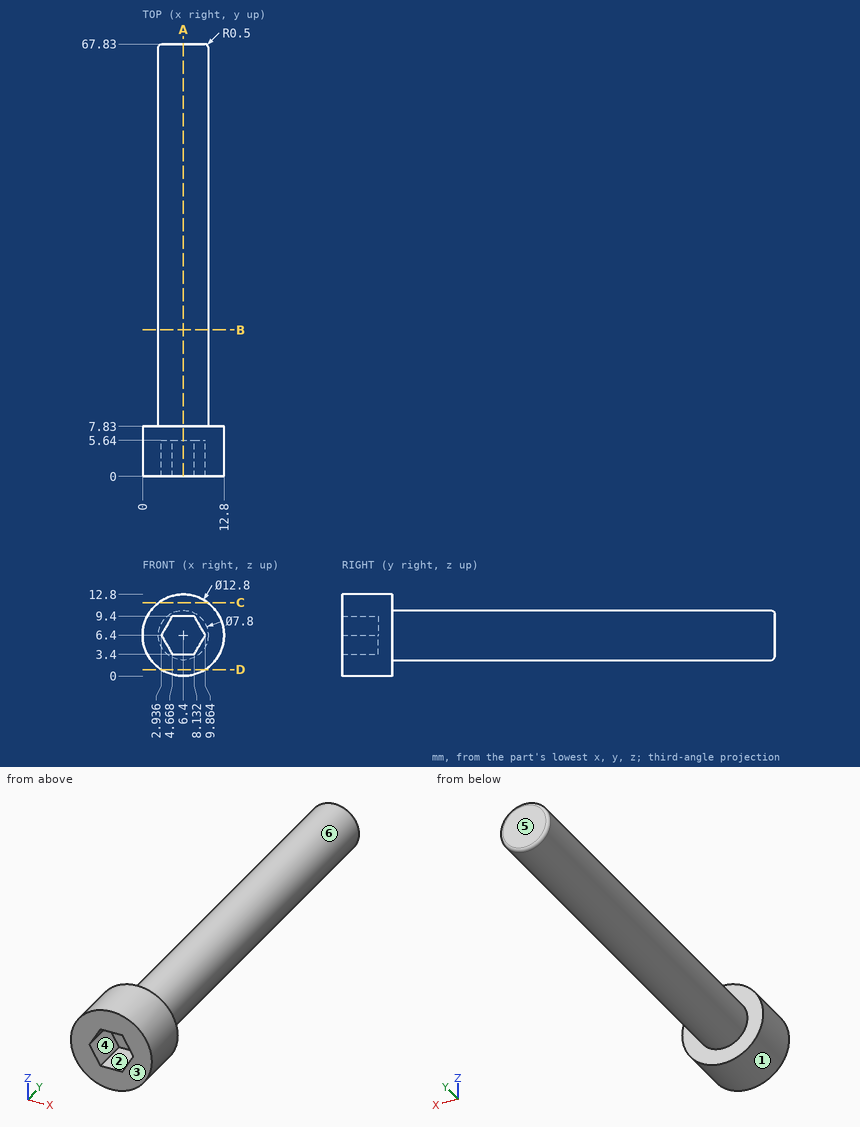
Answer from the drawing. Dimensions are ordinates in mm from the lowest x, y and z of the part. A direction names the side the tool comes from. Round coordinates to 2 decimals unless told otherwise and drop trailing zeros. Loops run counter-clockwise (first coordinate to the right, second up) from the corner with the lowest first, then second, coordinate; pieces in that order, holes last.
1) Consider line 1 (Y direction, x = 11.25, z = 6.5); line 2 (Z direction, x = 9.75, y = 5); line 3 (Y direction, x = 4.75, z = 6.5). Determine where each line is inside the solid, lowest interval first.
Outcome:
line 1: y = 0 to 7.83
line 2: z = 0.95 to 6.2, 6.6 to 11.85
line 3: y = 5.64 to 67.83
2) A cutting plane is placed at B-B on y = 23. Determine the outline of the cut face in (x, z).
Outcome:
outline: circle Ø7.8 at (6.4, 6.4)
3) A cutting plane is placed at D-D on z = 1. Determine the outline of the cut face in (x, y) (3 decimals), plus the area to 3 significant figures.
Outcome:
outline: (2.965, 0) - (9.835, 0) - (9.835, 7.83) - (2.965, 7.83) - close
area: 53.8 mm2
4) A cutting plane is placed at A-A on x = 6.4. Determine the outline of the cut face in (y, z).
Outcome:
outline: (0, 0) - (7.83, 0) - (7.83, 2.5) - (67.33, 2.5) arc R0.5 ccw to (67.83, 3) - (67.83, 9.8) arc R0.5 ccw to (67.33, 10.3) - (7.83, 10.3) - (7.83, 12.8) - (0, 12.8) - (0, 9.4) - (5.64, 9.4) - (5.64, 3.4) - (0, 3.4) - close
5) For the marked faces 5 and 6, determine the directions among +Z, -Z, +X, -X, +Y, -Y from which every point of the face is accessible in a straight line to the end or side of a thin tool.
Outcome:
face 5: +Z, -Z, +X, -X, +Y
face 6: +Y
6) Given P1, Ø2, axis at y = 56.5, z = 5, coming from the -X side, flat-ended and moving along its own axis, determine where the tip first touches the part or whether it passes through.
Outcome:
P1: stops at x = 2.52
7) A cutting plane is placed at C-C on z = 11.5. Determine the outline of the cut face in (x, y).
Outcome:
outline: (2.53, 0) - (10.27, 0) - (10.27, 7.83) - (2.53, 7.83) - close
8) For a pull along X with two mould halves and no side action, classify the marked faces 1, 2, 3 and 4 as released by +X, released by -X, zero draft, split by the parting line, or undercut.
Outcome:
face 1: split by the parting line
face 2: undercut
face 3: zero draft
face 4: undercut
